Geometry check sheet. Reference: the model listing, model coordinates, mm. A direction names the side the tool comes from. Round coordinates to 2 decimals unless told otherwise and drop trailing zeros. Write each loop counter-clockwise with the first axis right and the second up, starting at its lowest first coordinate (ties: lowest second). Pieces come first, ordered by that corner, then holes. Notation, with made-up numbers: (-9, 9.5) - (3, 9.5) arc R16 ccw to (3, 14.5) - close; hole circle Ø7 at (-20.5, -5.5). An arc over 180 degrees is marked (long way). Return JSON: item names as keys, results as strings. Group by question number.
from build123d import *

# Parameters (mm, degrees)
F1_DEPTH  = 50
F2_T      = -1.5
F4_DEPTH  = 48.5
F5_R      = 1
F6_DEPTH  = 10
F7_R      = 4
F8_DEPTH  = 6
F9_R      = 1
F10_DEPTH = 5


with BuildPart() as f1:
    # F0 (on Top) → F1 (new body)
    with BuildSketch(Plane.XY):
        with BuildLine():
            Line((-39.653846, -58.894231), (44.346154, -58.894231))
            ThreePointArc((44.346154, -58.894231), (46.467474, -58.015551), (47.346154, -55.894231))
            Line((47.346154, -55.894231), (47.346154, 60.105769))
            ThreePointArc((47.346154, 60.105769), (46.467474, 62.22709), (44.346154, 63.105769))
            Line((44.346154, 63.105769), (-39.653846, 63.105769))
            ThreePointArc((-39.653846, 63.105769), (-41.775166, 62.22709), (-42.653846, 60.105769))
            Line((-42.653846, 60.105769), (-42.653846, -55.894231))
            ThreePointArc((-42.653846, -55.894231), (-41.775166, -58.015551), (-39.653846, -58.894231))
        make_face()
    extrude(amount=F1_DEPTH)

    # F2
    f2_openings = [f1.faces().sort_by_distance(p)[0] for p in [
        (2.346154, 2.105769, 50),
    ]]
    offset(amount=F2_T, openings=f2_openings)

    # F3 (on face) → F4 (join)
    with BuildSketch(Plane.XY.offset(1.5)):
        with BuildLine():
            Line((45.846154, 61.605769), (38.846154, 61.605769))
            Line((38.846154, 61.605769), (38.846154, 56.605769))
            ThreePointArc((38.846154, 56.605769), (39.43194, 55.191556), (40.846154, 54.605769))
            Line((40.846154, 54.605769), (45.846154, 54.605769))
            Line((45.846154, 54.605769), (45.846154, 61.605769))
        make_face()
        with BuildLine():
            Line((-34.153846, 61.605769), (-41.153846, 61.605769))
            Line((-41.153846, 61.605769), (-41.153846, 54.605769))
            Line((-41.153846, 54.605769), (-36.153846, 54.605769))
            ThreePointArc((-36.153846, 54.605769), (-34.739633, 55.191556), (-34.153846, 56.605769))
            Line((-34.153846, 56.605769), (-34.153846, 61.605769))
        make_face()
        with BuildLine():
            Line((-36.153846, -50.394231), (-41.153846, -50.394231))
            Line((-41.153846, -50.394231), (-41.153846, -57.394231))
            Line((-41.153846, -57.394231), (-34.153846, -57.394231))
            Line((-34.153846, -57.394231), (-34.153846, -52.394231))
            ThreePointArc((-34.153846, -52.394231), (-34.739633, -50.980017), (-36.153846, -50.394231))
        make_face()
        with BuildLine():
            Line((45.846154, -50.394231), (40.846154, -50.394231))
            ThreePointArc((40.846154, -50.394231), (39.43194, -50.980017), (38.846154, -52.394231))
            Line((38.846154, -52.394231), (38.846154, -57.394231))
            Line((38.846154, -57.394231), (45.846154, -57.394231))
            Line((45.846154, -57.394231), (45.846154, -50.394231))
        make_face()
    extrude(amount=F4_DEPTH)

    # F5 (on face) → F6 (cut)
    with BuildSketch(Plane.XY.offset(50)):
        with Locations((42.846154, -54.394231)):
            Circle(F5_R)
        with Locations((-38.153846, -54.394231)):
            Circle(F5_R)
        with Locations((-38.153846, 58.605769)):
            Circle(F5_R)
        with Locations((42.846154, 58.605769)):
            Circle(F5_R)
    extrude(amount=-F6_DEPTH, mode=Mode.SUBTRACT)

    # F7 (on face) → F8 (join)
    with BuildSketch(Plane.XY.offset(1.5)):
        with Locations((29.346154, 44.605769)):
            Circle(F7_R)
        with Locations((-24.653846, -43.394231)):
            Circle(F7_R)
        with Locations((29.346154, -43.394231)):
            Circle(F7_R)
        with Locations((-24.653846, 44.605769)):
            Circle(F7_R)
    extrude(amount=F8_DEPTH)

    # F9 (on face) → F10 (cut)
    with BuildSketch(Plane.XY.offset(7.5)):
        with Locations((29.346154, 44.605769)):
            Circle(F9_R)
        with Locations((-24.653846, -43.394231)):
            Circle(F9_R)
        with Locations((29.346154, -43.394231)):
            Circle(F9_R)
        with Locations((-24.653846, 44.605769)):
            Circle(F9_R)
    extrude(amount=-F10_DEPTH, mode=Mode.SUBTRACT)


solid = f1.part
1. Section check D-D (z = 44.5). Enter the section's corners in (x, y), and give its area (3 significant figures).
2. Tool access check on faces 4 (the face through (-39, -50.394, 25)), 5 (the face through (46.44, -58.04, 24.65)). Record the directions out of +Z, -Z, +X, -X, +Y, -Y that give a thin tool (end or side, any length) a straight path to the whole face; none if there is none.
3. Mould release check, pull along X, two halves, no side actions. Record for faces 1 (the face through (47.346, 1, 25)), 2 (the face through (45.846, 1, 25)), 3 (the face through (-41.8, -57.99, 24.65)): pulls with the +X half, pulls with the -X half, needs draft (parallel to the pull), parting line crosses it, or undercut.
4. Section check A-A (z = 35). Enter the section's corners in (x, y).
5. Section check B-B (y = -11.5). Enter the section's corners in (x, z), and give its area (4 significant figures).
6. Material ranges on line 1 along Y through (x, z) = (14, 24); line 2 along X through (y, z) = (46.5, 45.5); line 3 along Y through (x, z) = (-36.5, 37), recorded low to high.
7. Depth check by flat-ended pin: pin 1 Ø3 at (x, y) = (-30.5, 46.5) entering from +Z; pin 2 Ø2.5 at (x, y) = (-26.5, 45) entering from +Z; pin 3 Ø1.8 at (x, y) = (-24.65, 44.61) entering from +Z. Enter the tip coordinate at first touch or a pass-through.
8. Section check C-C (x = 16). Enter the section's corners in (y, z), and give its area (4 significant figures).
Result sheet:
{
 "1": {"outline": "(-42.65, -55.89) arc R3 ccw to (-39.65, -58.89) - (44.35, -58.89) arc R3 ccw to (47.35, -55.89) - (47.35, 60.11) arc R3 ccw to (44.35, 63.11) - (-39.65, 63.11) arc R3 ccw to (-42.65, 60.11) - close; hole (-41.15, -50.39) - (-36.15, -50.39) arc R2 cw to (-34.15, -52.39) - (-34.15, -57.39) - (38.85, -57.39) - (38.85, -52.39) arc R2 cw to (40.85, -50.39) - (45.85, -50.39) - (45.85, 54.61) - (40.85, 54.61) arc R2 cw to (38.85, 56.61) - (38.85, 61.61) - (-34.15, 61.61) - (-34.15, 56.61) arc R2 cw to (-36.15, 54.61) - (-41.15, 54.61) - close; hole circle Ø2 at (-38.15, -54.39); hole circle Ø2 at (-38.15, 58.61); hole circle Ø2 at (42.85, -54.39); hole circle Ø2 at (42.85, 58.61)", "area": "799 mm²"},
 "2": {"face 4": "+Z", "face 5": "+Z, -Z, +X, -Y"},
 "3": {"face 1": "pulls with the +X half", "face 2": "undercut", "face 3": "pulls with the -X half"},
 "4": {"outline": "(-42.65, -55.89) arc R3 ccw to (-39.65, -58.89) - (44.35, -58.89) arc R3 ccw to (47.35, -55.89) - (47.35, 60.11) arc R3 ccw to (44.35, 63.11) - (-39.65, 63.11) arc R3 ccw to (-42.65, 60.11) - close; hole (-41.15, -50.39) - (-36.15, -50.39) arc R2 cw to (-34.15, -52.39) - (-34.15, -57.39) - (38.85, -57.39) - (38.85, -52.39) arc R2 cw to (40.85, -50.39) - (45.85, -50.39) - (45.85, 54.61) - (40.85, 54.61) arc R2 cw to (38.85, 56.61) - (38.85, 61.61) - (-34.15, 61.61) - (-34.15, 56.61) arc R2 cw to (-36.15, 54.61) - (-41.15, 54.61) - close"},
 "5": {"outline": "(-42.65, 0) - (47.35, 0) - (47.35, 50) - (45.85, 50) - (45.85, 1.5) - (-41.15, 1.5) - (-41.15, 50) - (-42.65, 50) - close", "area": "280.5 mm²"},
 "6": {"line 1": "y = -58.89 to -57.39, 61.61 to 63.11", "line 2": "x = -42.65 to -41.15, 45.85 to 47.35", "line 3": "y = -58.89 to -50.39, 54.61 to 63.11"},
 "7": {"pin 1": "stops at z = 1.5", "pin 2": "stops at z = 7.5", "pin 3": "stops at z = 2.5"},
 "8": {"outline": "(-58.89, 0) - (63.11, 0) - (63.11, 50) - (61.61, 50) - (61.61, 1.5) - (-57.39, 1.5) - (-57.39, 50) - (-58.89, 50) - close", "area": "328.5 mm²"}
}
